Autodesk Inventor part; units mm, degrees
ref_plane "YZ Plane" through (0, 0, 0) normal (1, 0, 0) x (0, 1, 0)
ref_plane "XZ Plane" through (0, 0, 0) normal (0, 1, 0) x (-1, 0, 0)
ref_plane "XY Plane" through (0, 0, 0) normal (0, 0, 1) x (1, 0, 0)
sketch "Sketch1" plane through (0, 0, 0) normal (0, 1, 0) x (-1, 0, 0)
  arc A0 (-159.7794, 702.6597) -> (-160.5669, 701.8721) centre (-159.7794, 701.8721) ccw
  line L0 (-155.7462, 702.6597) -> (-155.7462, 704.2667)
  line L1 (-155.7462, 704.2667) -> (-153.4941, 704.2667)
  line L2 (-153.4941, 704.2667) -> (-153.4941, 702.7805)
  line L3 (-153.4941, 702.7805) -> (-152.5972, 702.7805)
  arc A1 (-164.1836, 648.4268) -> (-160.5669, 657.8731) centre (-174.7114, 657.8731) ccw
  line L4 (-160.5669, 657.8731) -> (-160.5669, 701.8721)
  arc A2 (-160.1794, 645.8656) -> (-160.7583, 645.6139) centre (-160.1783, 645.0714) ccw
  arc A3 (-164.1836, 648.4268) -> (-160.7583, 645.6139) centre (-162.4137, 647.0901) ccw
  line L5 (-155.7462, 645.8656) -> (-155.7462, 644.7447)
  line L6 (-155.7462, 644.7447) -> (-153.4959, 644.7447)
  line L7 (-153.4959, 644.7447) -> (-153.4959, 645.7914)
  arc A4 (-143.0499, 641.0266) -> (-142.8493, 642.7649) centre (-143.1468, 641.9185) ccw
  line L8 (-163.0475, 641.9081) -> (-143.0499, 641.0266)
  arc A5 (-166.5264, 650.2868) -> (-163.0475, 641.9081) centre (-162.4021, 647.0877) ccw
  arc A6 (-166.5264, 650.2868) -> (-167.6429, 666.7468) centre (-174.8334, 657.9912) ccw
  line L9 (-167.6429, 666.7468) -> (-167.6429, 671.3153)
  arc A7 (-166.8471, 672.1213) -> (-167.6429, 671.3153) centre (-166.8257, 671.3043) ccw
  line L10 (-166.8471, 672.1213) -> (-166.0512, 672.1176)
  arc A8 (-165.304, 671.5825) -> (-166.0512, 672.1176) centre (-166.0579, 671.319) ccw
  line L11 (-165.304, 671.5825) -> (-164.5204, 669.4361)
  line L12 (-164.5204, 669.4361) -> (-164.4882, 669.3468)
  arc A9 (-164.4882, 669.3468) -> (-164.2374, 669.1723) centre (-164.2343, 669.4443) ccw
  line L13 (-164.2374, 669.1723) -> (-163.8302, 669.1723)
  arc A10 (-163.8326, 669.1723) -> (-163.5671, 669.4384) centre (-163.8364, 669.4416) ccw
  line L14 (-163.5671, 669.4384) -> (-163.5671, 706.0242)
  line L15 (-163.5671, 706.0242) -> (-163.5671, 706.0613)
  line L16 (-163.5671, 706.0613) -> (-147.5434, 708.8923)
  arc A11 (-147.5434, 708.8923) -> (-147.8025, 710.4755) centre (-147.5845, 709.6983) ccw
  line L17 (-147.8025, 710.4755) -> (-163.5671, 707.6952)
  line L18 (-163.5671, 707.6952) -> (-164.9603, 707.6952)
  line L19 (-164.9603, 707.6952) -> (-164.9605, 706.5472)
  arc A12 (-165.374, 706.3282) -> (-164.9605, 706.5472) centre (-165.23, 706.5562) ccw
  line L20 (-165.374, 706.3282) -> (-167.226, 707.3966)
  arc A13 (-167.6397, 708.1008) -> (-167.226, 707.3966) centre (-166.8384, 708.0979) ccw
  line L21 (-167.6397, 708.1008) -> (-167.6393, 713.6964)
  arc A14 (-166.8357, 714.5011) -> (-167.6393, 713.6964) centre (-166.8345, 713.6963) ccw
  line L22 (-166.8357, 714.5011) -> (-164.1567, 714.5011)
  arc A15 (-163.353, 713.6974) -> (-164.1567, 714.5011) centre (-164.1583, 713.6958) ccw
  line L23 (-163.353, 713.6974) -> (-163.353, 712.3579)
  line L24 (-163.353, 712.3579) -> (-165.4962, 711.98)
  line L25 (-165.4962, 711.98) -> (-165.4962, 711.7118)
  arc A16 (-165.4962, 711.7118) -> (-163.8213, 710.1096) centre (-163.8924, 711.7118) ccw
  line L26 (-163.8213, 710.1096) -> (-146.2918, 713.1784)
  arc A17 (-144.5878, 707.1017) -> (-146.2918, 713.1784) centre (-146.018, 709.9779) ccw
  arc A18 (-152.5972, 702.7805) -> (-152.2275, 702.8725) centre (-152.6033, 703.5935) ccw
  line L27 (-155.7462, 702.6597) -> (-155.7462, 700.1597)
  line L28 (-155.7462, 700.1597) -> (-156.9462, 700.1597)
  line L29 (-156.9462, 700.1597) -> (-157.7628, 702.6597)
  line L30 (-157.7628, 702.6597) -> (-159.7794, 702.6597)
  line L31 (-155.7462, 645.8656) -> (-155.7462, 647.8656)
  line L32 (-155.7462, 647.8656) -> (-157.3545, 645.8656)
  line L33 (-157.3545, 645.8656) -> (-160.1794, 645.8656)
  line L34 (-142.8493, 642.7649) -> (-152.5613, 645.7914)
  line L35 (-144.5878, 707.1017) -> (-152.2275, 702.8725)
  line L36 (-152.5613, 645.7914) -> (-153.4959, 645.7914)
  point P0 (-160.5669, 683.588)
  dimension "d2" = 43.999
  dimension "d3" = 3.0002
  dimension "d6" = 2.5
  dimension "d7" = 1.2
  dimension "d8" = 2
extrude "Extrusion1" add sketch "Sketch1" along normal blind 5.3
properties part number "raspDinClipmmv2"
Source: CAD feature listing. Evaluate the final solid. Frame: model axes, mm. A direction names the side the tool comes from. Round coordinates to 2 decimals unless told otherwise and drop trailing zeros. Loops run counter-clockwise (first coordinate to the right, second up) from the corner with the lowest first, then second, coordinate; pieces in that order, holes last. Notation, with made-up numbers: (-6, -15.75) -> (8, -15.75) arc R19 cw to (8, 10.25) -> close; hole circle Ø9 at (9.5, -18.5). An arc over 180 degrees is marked (long way). Answer as a JSON object with one key per item and string values. Group by question number.
Q1. Section query B-B (z = 673). Output: boundary loops of the cut face in (x, y), plus the area to 3 significant figures.
Q2. Mould query, pull axis Z, two halves, no side actions, for faces 1 (the flat face through (161, 5.3, 681)), 2 (the flat face through (153.189, 2.613, 641.474)), 3 (the flat face through (166.287, 2.613, 706.855)). Classes: pulls with the +Z half, pulls with the -Z half, needs draft (parallel to the pull), parting line crosses it, or undercut.
Q3. Ray query, line 1 (Z direction, x = 153, y = 4.9); line 2 (Z direction, x = 153.75, y = 2.5); line 3 (Z direction, x = 144, y = 4.8). Return the intervals inside material, ascending. Write a range as from..to.
Q4. Section query C-C (z = 654.5). Output: boundary loops of the cut face in (x, y).
Q5. Contact query for flat-ended pins moving along their axis: P1, Ø1.6, axis at x = 159, y = 2.5, coming from the -Z side; P2, Ø1.6, axis at y = 2, z = 704, coming from the +X side; P3, Ø2.5, axis at x = 159.5, y = 2, coming from the +Z side. Output: stop coordinate, or through.
Q6. Section query A-A (x = 150.5). Output: boundary loops of the cut face in (y, z) (3 decimals), plus the area to 3 significant figures.
Q7. Access query for faces 4 (the flat face through (163.353, 3, 713)), 5 (the flat face through (161, 0, 681)), 6 (the cylindrical face through (163.54, 2.61, 658.89)), 7 (the flat face through (164.41, 2.61, 712.17)), 8 (the flat face through (156, 3, 700.16)). Directions: +Z, -Z, +X, -X, +Y, -Y. A direction counts if a zero-diameter tool reaches every point of the face in a straight line with its end or side. Return the directions, or none.
Completed:
{
 "1": {"outline": "(160.57, 0) -> (163.57, 0) -> (163.57, 5.3) -> (160.57, 5.3) -> close", "area": "15.9 mm²"},
 "2": {"face 1": "needs draft", "face 2": "pulls with the -Z half", "face 3": "undercut"},
 "3": {"line 1": "641.47..645.79, 702.78..707.93, 709.56..712", "line 2": "641.5..644.74, 704.27..707.8, 709.43..711.87", "line 3": "641.07..643.12, 707.48..712.48"},
 "4": {"outline": "(160.97, 0) -> (164.05, 0) -> (164.05, 5.3) -> (160.97, 5.3) -> close"},
 "5": {"P1": "z = 641.69", "P2": "x = 163.57", "P3": "z = 711.08"},
 "6": {"outline": "(0, 641.355) -> (5.3, 641.355) -> (5.3, 645.149) -> (0, 645.149) -> close; (0, 703.829) -> (5.3, 703.829) -> (5.3, 708.37) -> (0, 708.37) -> close; (0, 710) -> (5.3, 710) -> (5.3, 712.442) -> (0, 712.442) -> close", "area": "57.1 mm²"},
 "7": {"face 4": "+Z, +Y, -Y", "face 5": "+Z, -Z, +X, -X, -Y", "face 6": "+X, +Y, -Y", "face 7": "+Y, -Y", "face 8": "-X, +Y, -Y"}
}
